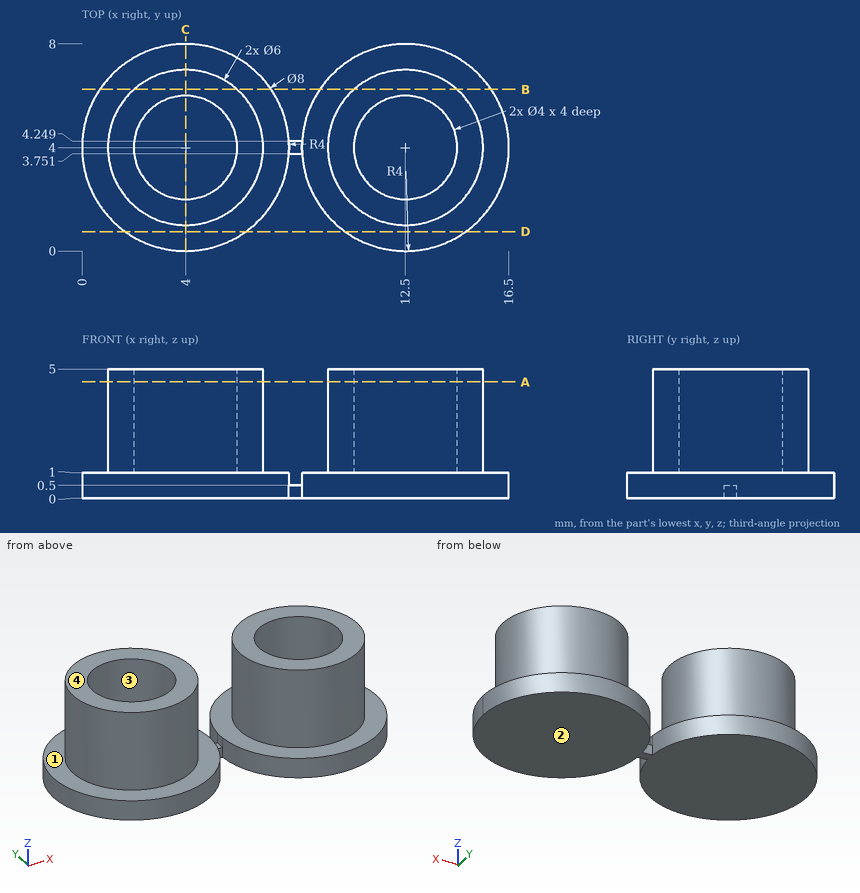
Source: three-view drawing plus pictorial views. Frame: mm from the lowest corner of the part. A direction names the side the tool comes from. Round coordinates to 2 decimals unless told otherwise and drop trailing zeros. Order: outer loops, then holes, each group sorted by start corner. A loop starts at its lowest first (then second) coordinate and runs counter-clockwise, first axis right, second up. Notation, with made-up numbers: M 27.25,77 L 63.25,77 A13 cw 63.25,101 Z; hole C 77,-11 d2. An arc over 180 degrees is marked long. One line per item, written item: value.
(1) Line query: probe 1 along Y at (x, z) = (4, 2.8); probe 2 along X at (y, z) = (3, 3.9); probe 3 along X at (y, z) = (2.75, 3.95). Output: solid intervals per line, ascending. Write a range as [from, to].
Result sheet:
probe 1: [1, 2], [6, 7]
probe 2: [1.17, 2.27], [5.73, 6.83], [9.67, 10.77], [14.23, 15.33]
probe 3: [1.27, 2.44], [5.56, 6.73], [9.77, 10.94], [14.06, 15.23]
(2) Cut plane B-B (y = 6.25). Return the cut outline in (x, z), and give its area (3 significant figures).
Result sheet:
outline: M 0.69,0 L 7.31,0 L 7.31,1 L 5.98,1 L 5.98,5 L 2.02,5 L 2.02,1 L 0.69,1 Z; M 9.19,0 L 15.81,0 L 15.81,1 L 14.48,1 L 14.48,5 L 10.52,5 L 10.52,1 L 9.19,1 Z
area: 45.0 mm2
(3) Reachability of the marked faces 3 and 4 from +Z, -Z, +X, -X, +Y, -Y: full face, straight path, thin tool, end or side. Return the list, or none.
Result sheet:
face 3: +Z
face 4: +Z, +X, -X, +Y, -Y
(4) Cut plane A-A (z = 4.5). Return the cut outline in (x, y), and give its area (3 significant figures).
Result sheet:
outline: C 4,4 d6; C 12.5,4 d6; hole C 4,4 d4; hole C 12.5,4 d4
area: 31.4 mm2
(5) Cut plane D-D (y = 0.75). Return the cut outline in (x, z).
Result sheet:
outline: M 1.67,0 L 6.33,0 L 6.33,1 L 1.67,1 Z; M 10.17,0 L 14.83,0 L 14.83,1 L 10.17,1 Z
(6) Pull-direction query (X, two-part tool) for the marked faces 1 and 2; classes: pulls with the +X half, pulls with the -X half, needs draft (parallel to the pull), parting line crosses it, or undercut.
Result sheet:
face 1: undercut
face 2: needs draft
(7) Pin query (flat end, axial travel): P1, Ø2.5, axis at x = 4, y = 4, coming from the +Z side; P2, Ø1.5, axis at x = 2, z = 2, coming from the -Y side; P3, Ø4, axis at x = 2.5, y = 3.5, coming from the +Z side. Return the tip coordinate at first contact, or that it passes through.
Result sheet:
P1: z = 1
P2: y = 1.27
P3: z = 5
(8) Cut plane C-C (x = 4). Return the cut outline in (y, z), and give its area (3 significant figures).
Result sheet:
outline: M 0,0 L 8,0 L 8,1 L 7,1 L 7,5 L 6,5 L 6,1 L 2,1 L 2,5 L 1,5 L 1,1 L 0,1 Z
area: 16.0 mm2
